```python
from build123d import *

# Parameters (mm, degrees)
SKETCH1_R           = 75
BOSS_EXTRUDE1_DEPTH = 10
SKETCH2_R           = 45
BOSS_EXTRUDE2_DEPTH = 10
SKETCH3_R           = 25
BOSS_EXTRUDE3_DEPTH = 44
FILLET1_R           = 20
SKETCH4_R           = 40
BOSS_EXTRUDE4_DEPTH = 10
SKETCH5_R           = 35
CUT_EXTRUDE1_DEPTH  = 20
SKETCH6_R           = 30
CUT_EXTRUDE2_DEPTH  = 2
SKETCH7_R           = 5
CUT_EXTRUDE3_DEPTH  = 124.878973196


with BuildPart() as part:
    # Sketch1 → Boss-Extrude1 (new body)
    with BuildSketch(Plane.XY):
        Circle(SKETCH1_R)
    extrude(amount=BOSS_EXTRUDE1_DEPTH)

    # Sketch2 → Boss-Extrude2 (add)
    with BuildSketch(Plane(origin=(0, 0, 0), x_dir=(-1, 0, 0), z_dir=(0, 0, -1))):
        Circle(SKETCH2_R)
    extrude(amount=BOSS_EXTRUDE2_DEPTH)

    # Sketch3 → Boss-Extrude3 (add)
    with BuildSketch(Plane(origin=(0, 0, -10), x_dir=(-1, 0, 0), z_dir=(0, 0, -1))):
        Circle(SKETCH3_R)
    extrude(amount=BOSS_EXTRUDE3_DEPTH)

    # Fillet1
    fillet1_edges = [part.edges().sort_by_distance(p)[0] for p in [
        (25, 0, -10),
    ]]
    fillet(fillet1_edges, radius=FILLET1_R - 0.0001)  # a hair under: the kernel refuses the full size

    # Sketch4 → Boss-Extrude4 (add)
    with BuildSketch(Plane.XY.offset(10)):
        Circle(SKETCH4_R)
    extrude(amount=BOSS_EXTRUDE4_DEPTH)

    # Sketch5 → Cut-Extrude1 (cut)
    with BuildSketch(Plane.XY.offset(20)):
        Circle(SKETCH5_R)
    extrude(amount=-CUT_EXTRUDE1_DEPTH, mode=Mode.SUBTRACT)

    # Sketch6 → Cut-Extrude2 (cut)
    with BuildSketch(Plane.XY):
        Circle(SKETCH6_R)
    extrude(amount=-CUT_EXTRUDE2_DEPTH, mode=Mode.SUBTRACT)

    # Sketch7 → Cut-Extrude3 (cut, through all)
    with BuildSketch(Plane.XY.offset(10)):
        with Locations((60, 0)):
            Circle(SKETCH7_R)
        with Locations((30, -51.961524227)):
            Circle(SKETCH7_R)
        with Locations((-30, -51.961524227)):
            Circle(SKETCH7_R)
        with Locations((-60, 0)):
            Circle(SKETCH7_R)
        with Locations((-30, 51.961524227)):
            Circle(SKETCH7_R)
        with Locations((30, 51.961524227)):
            Circle(SKETCH7_R)
    extrude(amount=-CUT_EXTRUDE3_DEPTH, mode=Mode.SUBTRACT)


solid = part.part
```
CAD build for the part. Positions are in the model's coordinates, mm. A direction names the side the tool comes from. Coordinates: 2 decimals unless noted, no trailing zeros. Order: outer loops, then holes, each group sorted by start corner. A loop starts at its lowest first (then second) coordinate and runs counter-clockwise, first axis right, second up. Notation, with made-up numbers: (39, 72) - (84, 72) arc R33 cw to (84, 102) - close; hole circle Ø10 at (76.25, 80.25). An arc over 180 degrees is marked (long way). Answer in a Markdown table with one row per item.
1. Pull direction Y, two halves, no side cores. Call faces 4 (the face through (0, 0, -2)), 5 (the face through (-20.765, -39.923, -4.93)), 6 (the face through (0, 0, -54)): +Y half, -Y half, draft (parallel to the pull), parting line (faces both ways), or undercut.
Answer:
| item | result |
|---|---|
| face 4 | undercut |
| face 5 | parting line |
| face 6 | draft |
2. Slice it at A-A, the plane y = 0. Give the number of separate pieces and of enclosed holes in the cut face, then the cut area to 3 significant figures.
Answer:
| item | result |
|---|---|
| separate pieces | 3 |
| enclosed holes | 0 |
| area | 3,850 mm² |
3. 3-axis set-ups, long thin cutter, end or side, ignore diameter. For faces 1 (the face through (32, -32, 10)), 2 (the face through (-33.7, -48.6, 5.1)), 3 (the face through (32, -32, 0)): which of +Z, -Z, +X, -X, +Y, -Y reach the whole face in a straight line?
Answer:
| item | result |
|---|---|
| face 1 | +Z |
| face 2 | +Z, -Z |
| face 3 | -Z |
4. Drill centre lines: L1, parallel to Y at x = -30, z = 3; L2, parallel to Z at x = -7, y = -45.5; L3, parallel to Y at x = -19, z = 15. Where is each one in solid material? Low to high. Write a range as from..to.
Answer:
| item | result |
|---|---|
| L1 | -68.74..-56.96, -46.96..-18.03, 18.03..46.96, 56.96..68.74 |
| L2 | 0..10 |
| L3 | -35.2..-29.39, 29.39..35.2 |
5. Slice it at C-C, the plane z = 8. List the corners of the cut face in (x, y), then the cut area to 3 significant figures.
Answer:
| item | result |
|---|---|
| outline | circle Ø150 at (0, 0); hole circle Ø10 at (-60, 0); hole circle Ø10 at (-30, -51.96); hole circle Ø70 at (0, 0); hole circle Ø10 at (-30, 51.96); hole circle Ø10 at (30, -51.96); hole circle Ø10 at (30, 51.96); hole circle Ø10 at (60, 0) |
| area | 13,400 mm² |
6. Slice it at B-B, the plane x = 60. List the corners of the cut face in (y, z), then the cut area to 3 significant figures.
Answer:
| item | result |
|---|---|
| outline | (-45, 0) - (-5, 0) - (-5, 10) - (-45, 10) - close; (5, 0) - (45, 0) - (45, 10) - (5, 10) - close |
| area | 800 mm² |
7. Flat gauge pins, fed straight in: P1, Ø12, axis at x = -15.5, z = -43, coming from the -Y side; P2, Ø16, axis at x = 30, y = 51.96, coming from the -Z side; P3, Ø4, axis at x = 50, y = -41, coming from the +Z side; P4, Ø6, axis at x = 32, z = -21.5, coming from the -Y side. Where does each tip first touch, or does it go through?
Answer:
| item | result |
|---|---|
| P1 | y = -23.12 |
| P2 | z = 0 |
| P3 | z = 10 |
| P4 | through |
